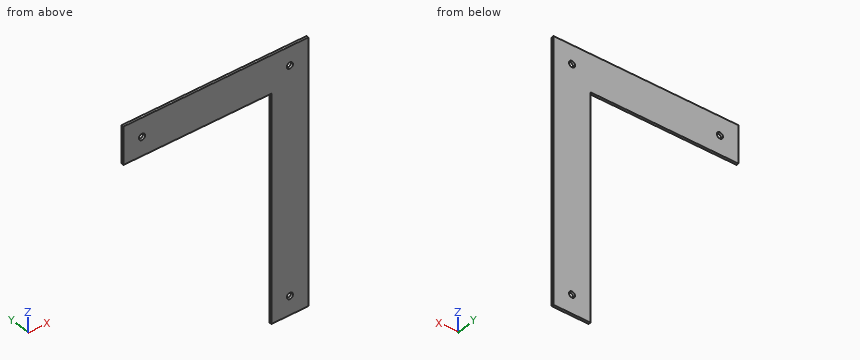
Autodesk Inventor part; units mm, degrees
ref_plane "YZ Plane" through (0, 0, 0) normal (1, 0, 0) x (0, 1, 0)
ref_plane "XZ Plane" through (0, 0, 0) normal (0, 1, 0) x (-1, 0, 0)
ref_plane "XY Plane" through (0, 0, 0) normal (0, 0, 1) x (1, 0, 0)
sketch "Sketch1" plane through (0, 0, 0) normal (0, 1, 0) x (-1, 0, 0)
  line L0 (-63.5, -88.9) -> (63.5, -88.9)
  line L1 (63.5, -88.9) -> (63.5, 88.9)
  line L2 (63.5, 88.9) -> (-63.5, 88.9)
  line L3 (-63.5, 88.9) -> (-63.5, -88.9)
  line L4 (-63.5, -88.9) -> (63.5, 88.9) construction
  line L5 (63.5, -88.9) -> (-63.5, 88.9) construction
  line L6 (63.5, -88.9) -> (-38.1, -88.9)
  line L7 (-38.1, -88.9) -> (-38.1, 63.5)
  line L8 (-38.1, 63.5) -> (63.5, 63.5)
  line L9 (63.5, 63.5) -> (63.5, -88.9)
  point P0 (0, 0)
  dimension "d0" = 127
  dimension "d1" = 177.8
  dimension "d2" = 101.6
  dimension "d3" = 152.4
extrude "Extrusion1" add sketch "Sketch1" along normal blind 1.5875 contours L3 L2 L1 L8 L7 L0
sketch "Sketch2" plane through (0, 1.5875, 0) normal (0, 1, 0) x (1, 0, 0)
  line L0 (-63.5, -63.5) -> (-63.5, -88.9)
  line L1 (-63.5, -88.9) -> (63.5, -88.9)
  line L2 (63.5, -88.9) -> (63.5, 88.9)
  line L3 (63.5, 88.9) -> (38.1, 88.9)
  line L4 (-63.5, -76.2) -> (63.5, -76.2) construction
  line L5 (50.8, 88.9) -> (50.8, -88.9) construction
  point P0 (0, 0)
  point P1 (-50.8, -76.2)
  point P2 (50.8, 76.2)
  point P3 (50.8, -76.2)
  dimension "d6" = 12.7
  dimension "d7" = 12.7
hole "Hole1" at (-50.8, 1.5875, 76.2) at (50.8, 1.5875, -76.2) at (50.8, 1.5875, 76.2) direction (0, -1, 0) diameter 4.191 end through all
properties part number "topLayer"
Geometry: final body of the model. Coordinates: model frame, mm. Round coordinates to 2 decimals unless told otherwise and drop trailing zeros. Loops run counter-clockwise (first coordinate to the right, second up) from the corner with the lowest first, then second, coordinate; pieces in that order, holes last.
Q1. Section D-D on x = 50.8. Return loops of the section in (y, z), plus the area to 3 significant figures.
Q2. Section B-B on x = -50.8. Return loops of the section in (y, z).
Q3. Section C-C on y = 1. Return loops of the section in (x, z).
Q4. Pin query (flat end, axial travel): P1, Ø0.5, axis at y = 0.5, z = 4.5, coming from the -X side; P2, Ø3.5, axis at x = 50.8, z = 76.2, coming from the -Y side; P3, Ø5, axis at x = -50.8, z = 76.2, coming from the +Y side. Return the tip coordinate at first contact, or that it passes through.
Q5. Material intervals for L1, parallel to X at y = 0.3, z = 76.2; L2, parallel to Z at x = 50.8, y = 0.75; L3, parallel to Z at x = -50.8, y = 0.6, sorted ascending.
Q6. Section A-A on z = -76.2. Return loops of the section in (x, y).
Evaluation:
1. outline: (0, -88.9) - (1.59, -88.9) - (1.59, -78.3) - (0, -78.3) - close; (0, -74.1) - (1.59, -74.1) - (1.59, 74.1) - (0, 74.1) - close; (0, 78.3) - (1.59, 78.3) - (1.59, 88.9) - (0, 88.9) - close
1. area: 269 mm2
2. outline: (0, 63.5) - (1.59, 63.5) - (1.59, 74.1) - (0, 74.1) - close; (0, 78.3) - (1.59, 78.3) - (1.59, 88.9) - (0, 88.9) - close
3. outline: (-63.5, 63.5) - (38.1, 63.5) - (38.1, -88.9) - (63.5, -88.9) - (63.5, 88.9) - (-63.5, 88.9) - close; hole circle Ø4.19 at (-50.8, 76.2); hole circle Ø4.19 at (50.8, -76.2); hole circle Ø4.19 at (50.8, 76.2)
4. P1: stops at x = 38.1
4. P2: passes through
4. P3: stops at y = 1.59
5. L1: x = -63.5 to -52.9, -48.7 to 48.7, 52.9 to 63.5
5. L2: z = -88.9 to -78.3, -74.1 to 74.1, 78.3 to 88.9
5. L3: z = 63.5 to 74.1, 78.3 to 88.9
6. outline: (38.1, 0) - (48.7, 0) - (48.7, 1.59) - (38.1, 1.59) - close; (52.9, 0) - (63.5, 0) - (63.5, 1.59) - (52.9, 1.59) - close
